Input: part model. Units: mm. Frame: model coordinates. Face numbers are marked on the shaded views. A direction names the side the tool comes from. Round coordinates to 2 decimals unless told otherwise and drop trailing zeros. Write each loop counter-clockwise with the first axis right and the second up, starting at its lowest first coordinate (ties: lowest second). Pieces come first, ordered by that corner, then holes. Notation, with made-up numbers: (-37, 52.25) - (-15, 52.25) arc R16 ccw to (-15, 75.25) - close; hole circle Ø8 at (-35.75, 22). An arc over 180 degrees is marked (long way). Use one line per item in the form item = value.
```python
from build123d import *

# Parameters (mm, degrees)
SKETCH_1_W           = 20
SKETCH_1_H           = 10
SKETCH_1_R           = 1.6
EXTRUDE_1_DEPTH      = 2
EXTRUDE_2_DEPTH      = 5
EXTRUDE_2_DEPTH_BACK = 25
FILLET_1_R           = 5
SKETCH_3_R           = 1.55
CUT_EXTRUDE_1_DEPTH  = 10
SKETCH_4_W           = 1.4
SKETCH_4_H           = 7
EXTRUDE_3_DEPTH      = 2


with BuildPart() as part:
    # 草图1 → 凸台-拉伸1 (new body)
    with BuildSketch(Plane(origin=(0, 0, 0), x_dir=(1, 0, 0), z_dir=(0, 1, 0))):
        Rectangle(SKETCH_1_W, SKETCH_1_H)
        with Locations(Location((-4.5, 1.5, 0), (0, 0, 270))):
            Circle(SKETCH_1_R, mode=Mode.SUBTRACT)
        with Locations(Location((4.5, 1.5, 0), (0, 0, 90))):
            Circle(SKETCH_1_R, mode=Mode.SUBTRACT)
    extrude(amount=EXTRUDE_1_DEPTH)

    # 草图2 → 凸台-拉伸2 (add, two sides: drawn at the far end of the back side and taken through both)
    with BuildSketch(Plane(origin=(10, 0, 0), x_dir=(0, 0, -1), z_dir=(1, 0, 0)).offset(-EXTRUDE_2_DEPTH_BACK)):
        Polygon((-5, 0), (-3, 0), (-37.93939209, 60.656729885), (-39.93939209, 60.656729885), align=None)
    extrude(amount=EXTRUDE_2_DEPTH + EXTRUDE_2_DEPTH_BACK)

    # 圆角1
    # the kernel refuses this fillet: 5 mm, written as the material it takes off along each edge
    with BuildSketch(Plane(origin=(-15, 60.656729885, 25.43939209), x_dir=(1, 0, 0), z_dir=(0, 0, 1)), Plane(origin=(15, 60.656729885, 25.43939209), x_dir=(0, -1, 0), z_dir=(0, 0, 1))) as fillet_1_piece_1:
        with BuildLine():
            CenterArc((FILLET_1_R, -FILLET_1_R), FILLET_1_R, 90, 90)
            Line((0, -FILLET_1_R), (0, 0))
            Line((0, 0), (FILLET_1_R, 0))
        make_face()
    extrude(amount=27, mode=Mode.SUBTRACT)

    # 草图3 → 切除-拉伸1 (cut)
    with BuildSketch(Plane(origin=(0, -1.297536287, 2.252595233), x_dir=(-1, 0, 0), z_dir=(0, 0.4991341727193529, -0.8665247126445773))):
        with Locations(Location((-12, 67.497402518, 0), (0, 0, 90))):
            Circle(SKETCH_3_R)
        with Locations(Location((12, 67.497402518, 0), (0, 0, 90))):
            Circle(SKETCH_3_R)
        with BuildLine():
            Line((12, 24.497402518), (12, 4.497402518))
            Line((12, 4.497402518), (-12, 4.497402518))
            Line((-12, 4.497402518), (-12, 24.497402518))
            add(Edge.make_bspline(
                [(-12, 24.497402518), (0, 35.211223002), (12, 24.497402518)],
                knots=[0, 0, 0, 1, 1, 1], degree=2))
        make_face()
    extrude(amount=-CUT_EXTRUDE_1_DEPTH, mode=Mode.SUBTRACT)

    # 草图4 → 凸台-拉伸3 (add)
    with BuildSketch(Plane(origin=(0, -1.297536287, 2.252595233), x_dir=(-1, 0, 0), z_dir=(0, 0.4991341727193529, -0.8665247126445773))):
        with Locations((0, 67.997402518)):
            Rectangle(SKETCH_4_W, SKETCH_4_H)
    extrude(amount=EXTRUDE_3_DEPTH)


solid = part.part
```
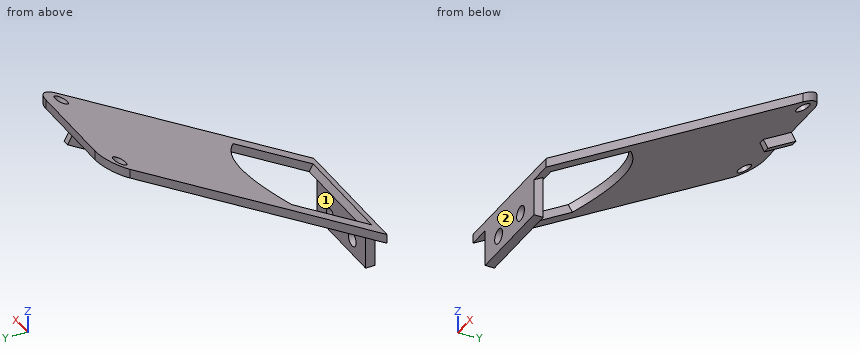
(1) Cut plane B-B on y = 14. Output: boundary loops of the cut face in (x, z), then the cut area to 3 significant figures.
Derived:
outline = (-15, 11.06) - (-12, 11.06) - (-12, 13.06) - (-15, 13.06) - close; (12, 11.06) - (15, 11.06) - (15, 13.06) - (12, 13.06) - close
area = 12.0 mm^2
(2) Material intervals for L1, parallel to X at y = 0.85, z = -1.5; L2, parallel to X at y = 12, z = 11.5; L3, parallel to Y at x = 3.5, z = 0.5, sorted ascending.
Derived:
L1 = -10 to -6.1, -2.9 to 2.9, 6.1 to 10
L2 = -15 to -12, 12 to 15
L3 = 0 to 2
(3) First-contact query: pin 1 Ø2.5 at (y, z) = (58, 35.5) entering from +X; pin 2 Ø5.5 at (y, z) = (10.5, 12) entering from -X; pin 3 Ø7.5 at (x, z) = (-2, 1.5) entering from +Y; pin 4 Ø4 at (y, z) = (60, 35) entering from -X. Flat tips, straight axial feed; report the tip coordinate or a pass-through.
Derived:
pin_1 = 14.88
pin_2 = -15
pin_3 = 2.6
pin_4 = -0.7
(4) Cut plane C-C on x = 4.5. Count the separate pieces of the cut face and the enclosed holes in it, then the cut area to 3 significant figures.
Derived:
separate_pieces = 3
enclosed_holes = 0
area = 89.4 mm^2
(5) Cut plane D-D on y = 27.5. Output: boundary loops of the cut face in (x, z), then the cut area to 3 significant figures.
Derived:
outline = (-15, 18.84) - (15, 18.84) - (15, 20.84) - (-15, 20.84) - close
area = 60.0 mm^2
(6) Access query for the marked faces 1 and 2. Directions: +Z, -Z, +X, -X, +Y, -Y. A direction counts if a zero-diameter tool reaches every point of the face in a straight line with its end or side. Return the directions, or none.
Derived:
face_1 = -Z, +X, -X, +Y
face_2 = +Z, -Z, +X, -X, -Y
(7) Cut plane A-A on z = -1.5. Output: boundary loops of the cut face in (x, y).
Derived:
outline = (-10, 0) - (-6.1, 0) - (-6.1, 2) - (-10, 2) - close; (-2.9, 0) - (2.9, 0) - (2.9, 2) - (-2.9, 2) - close; (6.1, 0) - (10, 0) - (10, 2) - (6.1, 2) - close
